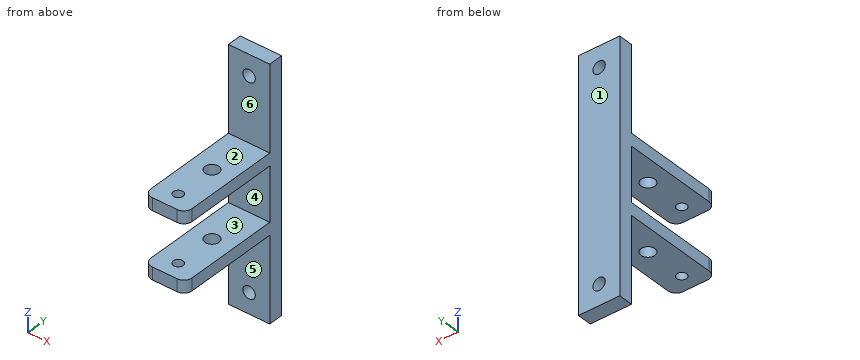
Autodesk Inventor part; units mm, degrees
ref_plane "YZ Plane" through (0, 0, 0) normal (1, 0, 0) x (0, 1, 0)
ref_plane "XZ Plane" through (0, 0, 0) normal (0, 1, 0) x (-1, 0, 0)
ref_plane "XY Plane" through (0, 0, 0) normal (0, 0, 1) x (1, 0, 0)
sketch "Szkic1" plane through (0, 0, 0) normal (0, 1, 0) x (-1, 0, 0)
  line L0 (-5, 30) -> (5, 30)
  line L1 (5, 30) -> (5, -30)
  line L2 (5, -30) -> (-5, -30)
  line L3 (-5, -30) -> (-5, 30)
  line L4 (-5, 30) -> (5, -30) construction
  line L5 (5, 30) -> (-5, -30) construction
  circle A0 centre (0, 25) radius 1.5
  circle A1 centre (0, -25) radius 1.5
  point P0 (0, 0)
  dimension "d0" = 10
  dimension "d1" = 60
  dimension "d2" = 50
  dimension "d3" = 5
  dimension "d4" = 5
  dimension "d5" = 3
  dimension "d6" = 3
extrude "Wyciągnięcie proste1" add sketch "Szkic1" along normal blind 3.5
sketch "Szkic2" plane through (0, 0, 0) normal (0, -1, 0) x (1, 0, 0)
  line L0 (5, 30) -> (5, -30)
  line L1 (-5, -9.5) -> (5, -9.5)
  line L2 (5, -9.5) -> (5, -6.5)
  line L3 (5, -6.5) -> (-5, -6.5)
  line L4 (-5, -6.5) -> (-5, -9.5)
  line L5 (-5, 6.5) -> (5, 6.5)
  line L6 (5, 6.5) -> (5, 9.5)
  line L7 (5, 9.5) -> (-5, 9.5)
  line L8 (-5, 9.5) -> (-5, 6.5)
  line L9 (-5, 30) -> (-5, -30)
  point P0 (0, 0)
  dimension "d9" = 3
  dimension "d10" = 3
  dimension "d11" = 13
  dimension "d12" = 6.5
extrude "Wyciągnięcie proste2" add sketch "Szkic2" along normal blind 25 contours L0 L5 L8 L7 | L0 L1 L4 L3
fillet "Zaokrąglenie1" radius 2 4 edges at (5, -25, -8) (-5, -25, -8) (5, -25, 8) (-5, -25, 8)
sketch "Szkic3" plane through (-5, 0, 9.5) normal (0, 0, 1) x (1, 0, 0)
  line L0 (0, 0) -> (0, -23)
  line L1 (8, -25) -> (2, -25)
  point P0 (5, 0)
  point P1 (5, -21)
  point P2 (5, -11)
  dimension "d16" = 10
  dimension "d17" = 5
  dimension "d18" = 4
hole "Otwór1" at (0, -11, 9.5) direction (0, 0, -1) diameter 3.4 end through all
hole "Otwór2" at (0, -21, 9.5) direction (0, 0, -1) diameter 2.4 end through all
equation "\"d10\" = d9"
Verification items for the finished model (mm, model axes). Face numbers are marked on the shaded views. A direction names the side the tool comes from. Give positions to 0.01 mm unless a question says otherwise; leave off trailing zeros. Loops run counter-clockwise (first coordinate to the right, second up) from the corner with the lowest first, then second, coordinate; pieces in that order, holes last.
1. Set-up check for the marked faces 4, 5 and 6: record each of +Z, -Z, +X, -X, +Y, -Y from which the full face is reachable in a straight line by a thin tool's end or side.
2. Section check D-D, the plane x = 0. Count the separate pieces of the cut face and the enclosed holes in it, then the cut area to 3 significant figures.
3. Thickness scan on line 1 (Z direction, x = 0, y = 2.2); line 2 (Y direction, x = 0, z = -8.3); line 3 (Z direction, x = -4.5, y = -5.25). Record the ranges inside material, lowest first.
4. Section check C-C, the plane y = -5.5. Enter the section's corners in (x, z).
5. Section check A-A, the plane z = -25. Enter the section's corners in (x, y).
6. Section check B-B, the plane y = -21. Enter the section's corners in (x, z), then the cut area to 3 significant figures.
7. Mould release check, pull along Z, two halves, no side actions. Record for the marked faces 1, 2 and 3: released by +Z, released by -Z, zero draft, split by the parting line, or undercut.
8. Go/stop test with flat-tipped pins: pin 1 Ø2 at (x, y) = (0, -11) entering from +Z; pin 2 Ø3 at (x, z) = (-1.5, 0.5) entering from -Y; pin 3 Ø6 at (x, y) = (1.5, -15) entering from -Z; pin 4 Ø5 at (x, y) = (0.5, -7) entering from +Z. Record where each tip stops, or that it passes through.
Geometry says:
1. face 4: +X, -X, -Y
1. face 5: -Z, +X, -X, -Y
1. face 6: +Z, +X, -X, -Y
2. separate pieces: 7
2. enclosed holes: 0
2. area: 304 mm2
3. line 1: z = -30 to -26.5, -23.5 to 23.5, 26.5 to 30
3. line 2: y = -25 to -22.2, -19.8 to -12.7, -9.3 to 3.5
3. line 3: z = -9.5 to -6.5, 6.5 to 9.5
4. outline: (-5, -9.5) - (5, -9.5) - (5, -6.5) - (-5, -6.5) - close; (-5, 6.5) - (5, 6.5) - (5, 9.5) - (-5, 9.5) - close
5. outline: (-5, 0) - (-1.5, 0) - (-1.5, 3.5) - (-5, 3.5) - close; (1.5, 0) - (5, 0) - (5, 3.5) - (1.5, 3.5) - close
6. outline: (-5, -9.5) - (-1.2, -9.5) - (-1.2, -6.5) - (-5, -6.5) - close; (-5, 6.5) - (-1.2, 6.5) - (-1.2, 9.5) - (-5, 9.5) - close; (1.2, -9.5) - (5, -9.5) - (5, -6.5) - (1.2, -6.5) - close; (1.2, 6.5) - (5, 6.5) - (5, 9.5) - (1.2, 9.5) - close
6. area: 45.6 mm2
7. face 1: zero draft
7. face 2: released by +Z
7. face 3: undercut
8. pin 1: passes through
8. pin 2: stops at y = 0
8. pin 3: stops at z = -9.5
8. pin 4: stops at z = 9.5
